from build123d import *

# Parameters (mm, degrees)
F0_W     = 81.28
F0_H     = 132.08
F1_DEPTH = 2.54
F2_R     = 3.175
F5_DEPTH = 2.54
F4_R     = 3.81
F6_DEPTH = 2.54
F3_R     = 3.81
F7_DEPTH = 2.54


with BuildPart() as f1:
    # F0 (on Top) → F1 (new body)
    with BuildSketch(Plane.XY):
        with Locations((-118.42192, -3.005858)):
            Rectangle(F0_W, F0_H)
    extrude(amount=F1_DEPTH)

    # F2 (on face) → F5 (cut)
    with BuildSketch(Plane.XY.offset(2.54)):
        with Locations((-118.42192, 34.752253)):
            Circle(F2_R)
    extrude(amount=-F5_DEPTH, mode=Mode.SUBTRACT)

    # F4 (on face) → F6 (cut)
    with BuildSketch(Plane.XY.offset(2.54)):
        with Locations((-118.42192, -23.734093)):
            Circle(F4_R)
    extrude(amount=-F6_DEPTH, mode=Mode.SUBTRACT)

    # F3 (on face) → F7 (cut)
    with BuildSketch(Plane.XY.offset(2.54)):
        with Locations((-118.42192, 9.941366)):
            Circle(F3_R)
    extrude(amount=-F7_DEPTH, mode=Mode.SUBTRACT)


solid = f1.part
Read the model definition and answer for the solid it produces. Units are mm, in the model's axes. Coordinates: 2 decimals unless noted, no trailing zeros. Order: outer loops, then holes, each group sorted by start corner. A loop starts at its lowest first (then second) coordinate and runs counter-clockwise, first axis right, second up. Notation, with made-up numbers: M -17,51 L 15,51 A13 cw 15,70 Z; hole C 19,79 d8. An arc over 180 degrees is marked long. Put each result on its own line as item: value. Start each with the question number.
Item 1: Section A-A, the plane y = -25 is taken. Determine the outline of the cut face in (x, z).
Item 2: The mould has two halves that part along Y. Classify faces 1 (the face through (-122.23, 10.11, 1.29)), 2 (the face through (-119, -2, 0)), 3 (the face through (-119, -69.046, 1)): +Y half, -Y half, draft (parallel to the pull), parting line (faces both ways), or undercut.
Item 3: Consider probe 1 along Y at (x, z) = (-115, 0.45); probe 2 along Y at (x, z) = (-116, 2.3); probe 3 along X at (y, z) = (7, 1.5). Determine where each line is inside the solid, lowest interval first. Write a range as [from, to].
Computed:
1. outline: M -159.06,0 L -122.02,0 L -122.02,2.54 L -159.06,2.54 Z; M -114.83,0 L -77.78,0 L -77.78,2.54 L -114.83,2.54 Z
2. face 1: undercut
2. face 2: draft
2. face 3: -Y half
3. probe 1: y = [-69.05, -25.41], [-22.06, 8.27], [11.62, 63.03]
3. probe 2: y = [-69.05, -26.68], [-20.79, 7], [12.88, 32.7], [36.81, 63.03]
3. probe 3: x = [-159.06, -120.84], [-116, -77.78]
